Geometry: final body of the model. Coordinates: model frame, mm. A direction names the side the tool comes from. Give positions to 0.01 mm unless a question says otherwise; leave off trailing zeros. Order: outer loops, then holes, each group sorted by start corner. A loop starts at its lowest first (then second) coordinate and runs counter-clockwise, first axis right, second up. Notation, with made-up numbers: (64.25, 83) - (121.25, 83) arc R18 ccw to (121.25, 90) - close; hole circle Ø2 at (60.25, 71.5). An arc over 180 degrees is marked (long way). Use one line per item in the form item = value.
Autodesk Inventor part; units mm, degrees
ref_plane "YZ Plane" through (0, 0, 0) normal (1, 0, 0) x (0, 1, 0)
ref_plane "XZ Plane" through (0, 0, 0) normal (0, 1, 0) x (-1, 0, 0)
ref_plane "XY Plane" through (0, 0, 0) normal (0, 0, 1) x (1, 0, 0)
sketch "Эскиз1" plane through (0, 0, 0) normal (0, 1, 0) x (-1, 0, 0)
  line L0 (-2.5, 4) -> (-2.5, 0)
  line L1 (-5, 0) -> (-2.5, 0)
  line L2 (-5, 0) -> (-3.9282, 4)
  line L3 (-2.5, 4) -> (-3.9282, 4)
  line L4 (0, 0) -> (0, 7.6417) construction
revolve "Вращение1" add sketch "Эскиз1" angle 360 about axis through (0, 0, 0) along (0, 0, 1)
sketch "Эскиз2" plane through (0, 0, 0) normal (0, 1, 0) x (-1, 0, 0)
  line L0 (-6.7216, 8.8894) -> (-10.15, 5.7727)
  line L1 (-5, 0) -> (-10.1175, 4.2646)
  line L2 (-3.9282, 4) -> (-5.0816, 8.4029)
  arc A0 (-5.0816, 8.4029) -> (-6.7216, 8.8894) centre (-6.049, 8.1495) ccw
  arc A1 (-10.15, 5.7727) -> (-10.1175, 4.2646) centre (-9.4773, 5.0328) ccw
  line L3 (0, 0) -> (0, 6.5882) construction
  line L4 (6.7216, 8.8894) -> (10.15, 5.7727)
  line L5 (5, 0) -> (10.1175, 4.2646)
  line L6 (3.9282, 4) -> (5.0816, 8.4029)
  arc A2 (6.7216, 8.8894) -> (5.0816, 8.4029) centre (6.049, 8.1495) ccw
  arc A3 (10.1175, 4.2646) -> (10.15, 5.7727) centre (9.4773, 5.0328) ccw
  line L7 (-3.9282, 4) -> (-3.4282, 4)
  line L8 (-3.4282, 4) -> (-4.5049, 0)
  line L9 (-4.5049, 0) -> (-5, 0)
  line L10 (3.9282, 4) -> (3.4282, 4)
  line L11 (3.4282, 4) -> (4.5049, 0)
  line L12 (4.5049, 0) -> (5, 0)
extrude "Выдавливание1" add sketch "Эскиз2" along normal mid plane 2.5
fillet "Сопряжение1" radius 0.5 20 edges at (5.7646, -1.25, 9.1082) (8.4358, -1.25, 7.3311) (10.4771, -1.25, 5.0113) (7.5587, -1.25, 2.1323) (4.5049, -1.25, 6.2014) (10.4771, 1.25, 5.0113) (7.5587, 1.25, 2.1323) (5.7646, 1.25, 9.1082) (4.5049, 1.25, 6.2014) (8.4358, 1.25, 7.3311) (-5.7646, -1.25, 9.1082) (-8.4358, -1.25, 7.3311) (-10.4771, -1.25, 5.0113) (-7.5587, -1.25, 2.1323) (-4.5049, -1.25, 6.2014) (-5.7646, 1.25, 9.1082) (-8.4358, 1.25, 7.3311) (-10.4771, 1.25, 5.0113) (-7.5587, 1.25, 2.1323) (-4.5049, 1.25, 6.2014)
thread "Резьба1"
properties part number "Гайка-барашек М5"
(1) Ray query, line 1 along Z through (x, y) = (3, 1.5); line 2 along Y through (x, z) = (-6, 2); line 3 along X through (y, z) = (1, 5.5). Return the intervals inside material, ascending.
Computed values:
line_1 = 0 to 4
line_2 = -1.25 to 1.25
line_3 = -10.28 to -4.39, 4.39 to 10.28
(2) Contact query for flat-ended pins moving along their axis: pin 1 Ø1.5 at (x, z) = (-4, 5.5) entering from -Y; pin 2 Ø1 at (x, y) = (-0.5, 2.5) entering from +Z; pin 3 Ø4 at (x, y) = (0, 0) entering from -Z; pin 4 Ø1.9 at (x, z) = (-7, 2.5) entering from +Y. Output: stop coordinate, or through.
Computed values:
pin_1 = -1.25
pin_2 = 4
pin_3 = through
pin_4 = 1.25
(3) Cut plane A-A on x = 0. Output: boundary loops of the cut face in (y, z), plus the area to 3 significant figures.
Computed values:
outline = (-5, 0) - (-2.5, 0) - (-2.5, 4) - (-3.93, 4) - close; (2.5, 0) - (5, 0) - (3.93, 4) - (2.5, 4) - close
area = 15.7 mm²
(4) Reachability of faces 4 (the face through (4.497, -0.01, 6.171)), 5 (the face through (7, 1.25, 5)), 6 (the face through (4.65, -1.1, 6.2)) from +Z, -Z, +X, -X, +Y, -Y: full face, straight path, thin tool, end or side. Return the list, or none.
Computed values:
face_4 = +Z, +Y, -Y
face_5 = +Z, +X, +Y
face_6 = +Z, -Y
(5) Cut plane B-B on y = 0. Output: boundary loops of the cut face in (x, z), plus the area to 3 significant figures.
Computed values:
outline = (-10.15, 5.77) arc R1 ccw to (-10.12, 4.26) - (-5, 0) - (-2.5, 0) - (-2.5, 4) - (-3.93, 4) - (-5.08, 8.4) arc R1 ccw to (-6.72, 8.89) - close; (2.5, 0) - (5, 0) - (10.12, 4.26) arc R1 ccw to (10.15, 5.77) - (6.72, 8.89) arc R1 ccw to (5.08, 8.4) - (3.93, 4) - (2.5, 4) - close
area = 84.1 mm²
(6) Pull-direction query (X, two-part tool) for faces 1 (the face through (-4.642, 1.107, 6.133)), 2 (the face through (-7.474, -1.1, 2.247)), 3 (the face through (-0.08, 4.35, 2.42)); classes: released by +X, released by -X, zero draft, split by the parting line, or undercut.
Computed values:
face_1 = undercut
face_2 = released by -X
face_3 = split by the parting line
